Design review of the part shown in the three views and the two pictorial views. Dimensions are in mm from the part's minimum x, y and z. A direction names the side the tool comes from. Coordinates: 2 decimals unless noted, no trailing zeros. Loops run counter-clockwise (first coordinate to the right, second up) from the corner with the lowest first, then second, coordinate; pieces in that order, holes last.
Q1. Add section C-C on y = 5. Give the boundary of the cut face in (x, z).
Q2. Add section B-B on x = 26.5. Give the boundary of the cut face in (y, z), and give its area (3 significant figures).
Q3. Wall thickness on probe 1 along X at (y, z) = (7.5, 5.15); probe 2 along X at (y, z) = (8, 2.5); probe 3 along Z at (x, y) = (37, 9): over which ranges is each line inside the solid? List them lowest first.
Q4. Add section D-D on y = 9. Give the boundary of the cut face in (x, z).
Q5. Machinability: for the marked faces 3, 4 and 5, which of the approach directions +Z, -Z, +X, -X, +Y, -Y give a long, thin tool a straight path to every point of the face, cutting with its end or side? Answer none if there is none.
Q6. For P1, Ø5, axis at x = 27, y = 6.5, coming from the -Z side; P2, Ø7, axis at x = 5.15, z = 5.15, coming from the -Y side; P3, Ø2, axis at y = 5, z = 9.5, coming from the -X side; P4, Ø2, axis at x = 22.5, y = 7, coming from the +Z side, all flat-tipped, find the tip position at first contact; note any pin that passes through.
Q7. Draft analysis for pull direction X (two halves, no side actions). For the marked faces 1 and 2, state which applies: released by +X, released by -X, zero draft, split by the parting line, or undercut.
Q8. Add section A-A on z = 5.15. Give the boundary of the cut face in (x, y), and give its area (3 significant figures).
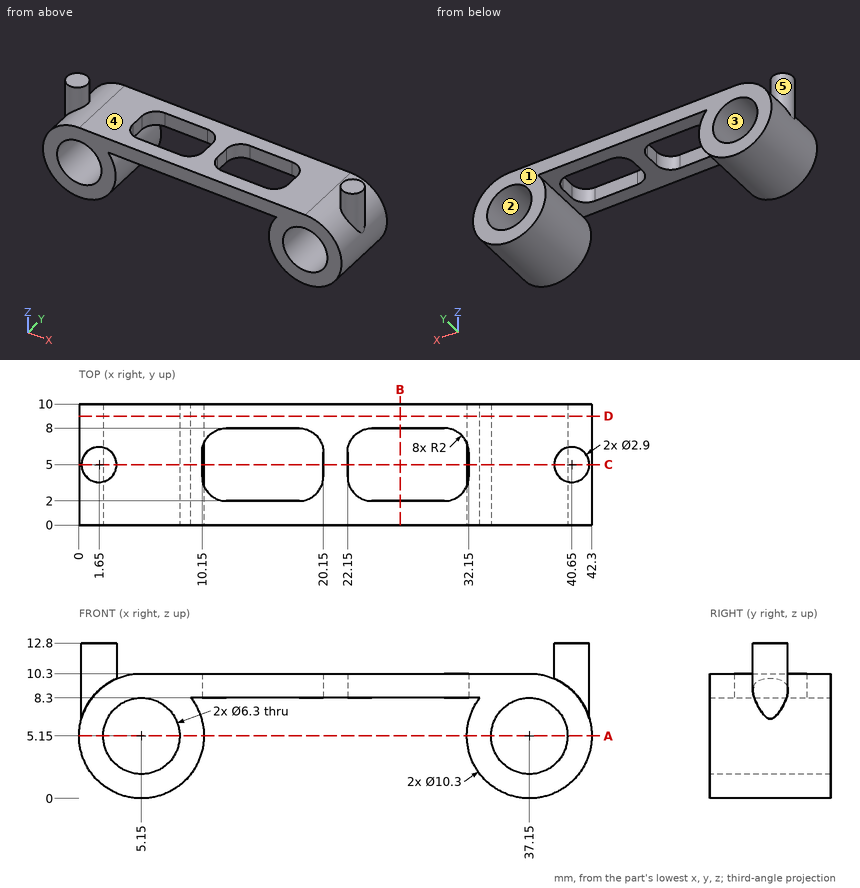
Entries:
1. outline: (0.2, 6.57) arc R5.15 ccw (long way) to (9.22, 8.3) - (10.15, 8.3) - (10.15, 10.3) - (5.15, 10.3) arc R5.15 ccw to (3.1, 9.87) - (3.1, 12.8) - (0.2, 12.8) - close; (20.15, 8.3) - (22.15, 8.3) - (22.15, 10.3) - (20.15, 10.3) - close; (32.15, 8.3) - (33.08, 8.3) arc R5.15 ccw (long way) to (42.1, 6.57) - (42.1, 12.8) - (39.2, 12.8) - (39.2, 9.87) arc R5.15 ccw to (37.15, 10.3) - (32.15, 10.3) - close; hole circle Ø6.3 at (5.15, 5.15); hole circle Ø6.3 at (37.15, 5.15)
2. outline: (0, 8.3) - (2, 8.3) - (2, 10.3) - (0, 10.3) - close; (8, 8.3) - (10, 8.3) - (10, 10.3) - (8, 10.3) - close
2. area: 8.00 mm2
3. probe 1: x = 0 to 2, 8.3 to 10.3, 32 to 34, 40.3 to 42.3
3. probe 2: x = 0.73 to 3.45, 6.85 to 9.57, 32.73 to 35.45, 38.85 to 41.57
3. probe 3: z = 0 to 2, 8.3 to 10.3
4. outline: (5.15, 10.3) arc R5.15 ccw (long way) to (9.22, 8.3) - (33.08, 8.3) arc R5.15 ccw (long way) to (37.15, 10.3) - close; hole circle Ø6.3 at (5.15, 5.15); hole circle Ø6.3 at (37.15, 5.15)
5. face 3: +Y, -Y
5. face 4: +Z, +Y, -Y
5. face 5: +Z
6. P1: stops at z = 8.3
6. P2: stops at y = 0
6. P3: stops at x = 0.2
6. P4: stops at z = 10.3
7. face 1: zero draft
7. face 2: undercut
8. outline: (0, 0) - (2, 0) - (2, 10) - (0, 10) - close; (8.3, 0) - (10.3, 0) - (10.3, 10) - (8.3, 10) - close; (32, 0) - (34, 0) - (34, 10) - (32, 10) - close; (40.3, 0) - (42.3, 0) - (42.3, 10) - (40.3, 10) - close
8. area: 80.0 mm2
